from build123d import *

# Parameters (mm, degrees)
SKETCH1_R                 = 70
BOSS_EXTRUDE1_DEPTH       = 10
SKETCH2_R                 = 65
BOSS_EXTRUDE2_DEPTH       = 3
BOSS_EXTRUDE3_DEPTH       = 5
M4X0_7_TAPPED_HOLE1_D     = 3.3
M4X0_7_TAPPED_HOLE1_DEPTH = 10.1
M4X0_7_TAPPED_HOLE1_TIP   = 0.991420021


with BuildPart() as part:
    # Sketch1 → Boss-Extrude1 (new body)
    with BuildSketch(Plane(origin=(0, 0, 0), x_dir=(1, 0, 0), z_dir=(0, 1, 0))):
        Circle(SKETCH1_R)
    extrude(amount=BOSS_EXTRUDE1_DEPTH)

    # Sketch2 → Boss-Extrude2 (add)
    with BuildSketch(Plane.XZ):
        Circle(SKETCH2_R)
    extrude(amount=BOSS_EXTRUDE2_DEPTH)

    # Sketch3 → Boss-Extrude3 (add, symmetric)
    with BuildSketch(Plane.XY):
        with BuildLine():
            Line((-25, 55), (-25, 5))
            Line((-25, 5), (-90, 5))
            Line((-90, 5), (-112.094257771, 43.204763027))
            ThreePointArc((-112.094257771, 43.204763027), (-75.29730578, 98.944673602), (-25, 55))
        make_face()
    extrude(amount=BOSS_EXTRUDE3_DEPTH, both=True)

    # M4x0.7 Tapped Hole1
    with Locations(Plane(origin=(0, 10, 0), x_dir=(1, 0, 0), z_dir=(0, 1, 0))):
        with Locations((4, 23.622), (51.244, 23.622), (51.244, -23.622), (4, -23.622)):
            Hole(M4X0_7_TAPPED_HOLE1_D / 2, depth=M4X0_7_TAPPED_HOLE1_DEPTH)
            with Locations((0, 0, -(M4X0_7_TAPPED_HOLE1_DEPTH + M4X0_7_TAPPED_HOLE1_TIP / 2))):  # 118° drill point
                Cone(0, M4X0_7_TAPPED_HOLE1_D / 2, M4X0_7_TAPPED_HOLE1_TIP, mode=Mode.SUBTRACT)


solid = part.part
Source: CAD feature listing. Evaluate the final solid. Frame: model axes, mm. A direction names the side the tool comes from. Give positions to 0.01 mm unless a question says otherwise; leave off trailing zeros. Order: outer loops, then holes, each group sorted by start corner. A loop starts at its lowest first (then second) coordinate and runs counter-clockwise, first axis right, second up. Notation, with made-up numbers: (71, 10.25) -> (90, 10.25) arc R19 ccw to (90, 39.25) -> close; hole circle Ø7 at (82, 29). An arc over 180 degrees is marked (long way). Write item = value, one per line.
Item 1: Section query A-A (x = 0). Output: boundary loops of the cut face in (y, z).
Check result:
outline = (-3, -65) -> (0, -65) -> (0, -70) -> (10, -70) -> (10, 70) -> (0, 70) -> (0, 65) -> (-3, 65) -> close
Item 2: Section query D-D (y = 80.5). Output: boundary loops of the cut face in (x, z), then the cut area to 3 significant figures.
Check result:
outline = (-105.63, -5) -> (-33.06, -5) -> (-33.06, 5) -> (-105.63, 5) -> close
area = 726 mm²
Item 3: Section query C-C (z = 0). Output: boundary loops of the cut face in (x, y), then the cut area to 3 significant figures.
Check result:
outline = (-112.09, 43.2) -> (-90, 5) -> (-70, 5) -> (-70, 0) -> (-65, 0) -> (-65, -3) -> (65, -3) -> (65, 0) -> (70, 0) -> (70, 10) -> (-25, 10) -> (-25, 55) arc R44.35 ccw (long way) to start
area = 8,600 mm²
Item 4: Ray query, probe 1 along Y at (x, z) = (45.5, 4.5); probe 2 along Z at (x, y) = (-85.5, 44); probe 3 along Z at (x, y) = (4, 7.5). Return the intervals inside material, ascending.
Check result:
probe_1 = -3 to 10
probe_2 = -5 to 5
probe_3 = -69.89 to -25.27, -21.97 to 21.97, 25.27 to 69.89
Item 5: Set-up query: faces 1 (the face through (-1, -3, 1)), 2 (the face through (-80, 5, 0)), 3 (the face through (62, -1.48, 19.52)), 4 (the face through (-25, 33, 0)). Return all of +Z, -Z, +X, -X, +Y, -Y with unobstructed straight access to the full face (end or side cutting, diameter ignored); none if empty.
Check result:
face_1 = +Z, -Z, +X, -X, -Y
face_2 = +Z, -Z, -X, -Y
face_3 = -Y
face_4 = +Z, -Z, +X, +Y
Item 6: Section query B-B (z = 16). Output: boundary loops of the cut face in (x, y), then the cut area to 3 significant figures.
Check result:
outline = (-68.15, 0) -> (-63, 0) -> (-63, -3) -> (63, -3) -> (63, 0) -> (68.15, 0) -> (68.15, 10) -> (-68.15, 10) -> close
area = 1,740 mm²
Item 7: Contact query for flat-ended pins moving along their axis: pin 1 (2 mm diameter, centred on x = 4, z = -23.622, fed in from +Y); pin 2 (1.5 mm diameter, centred on x = -66, z = 20.5, fed in from +Y); pin 3 (8 mm diameter, centred on x = -82.5, z = -1, fed in from -Y). Output: stop coordinate, or through.
Check result:
pin_1 = -0.49
pin_2 = 10
pin_3 = 5
